The model under review builds one solid part; all positions refer to its coordinate system, in mm. A direction names the side the tool comes from. Give positions to 0.01 mm unless a question says otherwise; leave off trailing zeros. Write each loop counter-clockwise with the first axis right and the second up, starting at its lowest first coordinate (ties: lowest second). Pieces come first, ordered by that corner, then holes. Notation, with made-up numbers: (-15.5, 50) -> (15.5, 50) arc R32 cw to (15.5, 85) -> close; hole circle Ø10 at (63, 26). An arc over 180 degrees is marked (long way). Use CSV: the item, a comma, the result in double quotes.
```python
from build123d import *

# Parameters (mm, degrees)
SKETCH1_W           = 48
SKETCH1_H           = 28
BOSS_EXTRUDE1_DEPTH = 1
SKETCH2_W           = 50
SKETCH2_H           = 30
BOSS_EXTRUDE2_DEPTH = 1
SKETCH3_R           = 3
BOSS_EXTRUDE3_DEPTH = 50
SKETCH4_R           = 1.8
CUT_EXTRUDE1_DEPTH  = 51
BOSS_EXTRUDE4_DEPTH = 5
CUT_EXTRUDE2_DEPTH  = 34


with BuildPart() as part:
    # Sketch1 → Boss-Extrude1 (new body)
    with BuildSketch(Plane(origin=(0, 0, 0), x_dir=(1, 0, 0), z_dir=(0, 1, 0))):
        Rectangle(SKETCH1_W, SKETCH1_H)
    extrude(amount=BOSS_EXTRUDE1_DEPTH)

    # Sketch2 → Boss-Extrude2 (add)
    with BuildSketch(Plane(origin=(0, 1, 0), x_dir=(1, 0, 0), z_dir=(0, 1, 0))):
        Rectangle(SKETCH2_W, SKETCH2_H)
    extrude(amount=BOSS_EXTRUDE2_DEPTH)

    # Sketch3 → Boss-Extrude3 (add)
    with BuildSketch(Plane.ZY.offset(25)):
        with Locations((-15, -1)):
            Circle(SKETCH3_R)
    extrude(amount=-BOSS_EXTRUDE3_DEPTH)

    # Sketch4 → Cut-Extrude1 (cut, through all)
    with BuildSketch(Plane.ZY.offset(25)):
        with Locations((-15, -1)):
            Circle(SKETCH4_R)
    extrude(amount=-CUT_EXTRUDE1_DEPTH, mode=Mode.SUBTRACT)

    # Sketch6 → Boss-Extrude4 (add, symmetric)
    with BuildSketch(Plane(origin=(0, 0, 0), x_dir=(0, 0, -1), z_dir=(1, 0, 0))):
        Polygon((-10.647346039, 2), (-11, 4), (-9, 4), (-9.352653961, 2), align=None)
    extrude(amount=BOSS_EXTRUDE4_DEPTH, both=True)

    # Sketch8 → Cut-Extrude2 (cut, through all)
    with BuildSketch(Plane.XY.offset(15)):
        with BuildLine():
            Line((3, 4), (5, 4))
            Line((5, 4), (5, 2))
            ThreePointArc((5, 2), (3.855631086, 2.855631086), (3, 4))
        make_face()
        with BuildLine():
            Line((-5, 4), (-5, 2))
            ThreePointArc((-5, 2), (-3.855631086, 2.855631086), (-3, 4))
            Line((-3, 4), (-5, 4))
        make_face()
    extrude(amount=-CUT_EXTRUDE2_DEPTH, mode=Mode.SUBTRACT)


solid = part.part
```
Q1. The part is to be moulded in two halves that separate along Y. For faces 1 (the flat face through (-0.3, 1.5, 15)), 2 (the flat face through (0, 4, 10)), 3 (the cylindrical face through (-0.35, -0.459, -13.283)), say which applies: pulls with the +Y half, pulls with the -Y half, needs draft (parallel to the pull), parting line crosses it, or undercut.
Derived:
face 1,"needs draft"
face 2,"pulls with the +Y half"
face 3,"undercut"
Q2. Consider section C-C (x = -2). Write out the cut boundary in (y, z).
Derived:
outline,"(0, -12.17) arc R3 ccw (long way) to (2, -15) -> (2, 9.35) -> (4, 9) -> (4, 11) -> (2, 10.65) -> (2, 15) -> (1, 15) -> (1, 14) -> (0, 14) -> close; hole circle Ø3.6 at (-1, -15)"
Q3. Consider section B-B (z = -6). Write out the cut boundary in (x, y), then the cut area to 3 significant figures.
Derived:
outline,"(-25, 1) -> (-24, 1) -> (-24, 0) -> (24, 0) -> (24, 1) -> (25, 1) -> (25, 2) -> (-25, 2) -> close"
area,"98.0 mm2"
Q4. To check wall thickness, follow probe 1 along Y at (x, z) = (7, -15); probe 2 along Z at (x, y) = (22, 0.5); probe 3 along Z at (x, y) = (17.5, -1.5). State the ranges of each line that lie inside material, in increasing order.
Derived:
probe 1,"y = -4 to -2.8, 0.8 to 2"
probe 2,"z = -17.6 to -15.99, -14.01 to 14"
probe 3,"z = -17.96 to -16.73, -13.27 to -12.04"
Q5. Consider section A-A (x = 7). Write out the cut boundary in (y, z).
Derived:
outline,"(0, -12.17) arc R3 ccw (long way) to (2, -15) -> (2, 15) -> (1, 15) -> (1, 14) -> (0, 14) -> close; hole circle Ø3.6 at (-1, -15)"
Q6. Machinability: for faces 4 (the flat face through (-0.3, 0.5, 14)), 5 (the cylindrical face through (-3.87, 2.84, 10.01)), which of the approach directions +Z, -Z, +X, -X, +Y, -Y give a long, thin tool a straight path to every point of the face, cutting with its end or side? Answer none if there is none.
Derived:
face 4,"+Z, +X, -X, -Y"
face 5,"+Z, -Z, -X, +Y"
Q7. Insertion check: pin 1 (9 mm diameter, centred on x = -3, z = 1, fed in from +Y); pin 2 (14 mm diameter, centred on x = 9, z = 3.5, fed in from -Y); pin 3 (3 mm diameter, centred on y = -1, z = -15, fed in from +X); pin 4 (0.8 mm diameter, centred on y = 0.5, z = -2.5, fed in from -X). Each pin has a flat end and moves straight along its axis. Give the tip position at first contact, or say it passes through.
Derived:
pin 1,"stops at y = 2"
pin 2,"stops at y = 0"
pin 3,"passes through"
pin 4,"stops at x = -24"
